```python
from build123d import *

# Parameters (mm, degrees)
F0_W     = 505
F0_H     = 250
F1_DEPTH = 40
F2_W     = 70
F2_H     = 20
F3_DEPTH = 3
F4_R     = 5
F5_DEPTH = 110


with BuildPart() as f1:
    # F0 (on Top) → F1 (new body)
    with BuildSketch(Plane.XY):
        Rectangle(F0_W, F0_H)
    extrude(amount=F1_DEPTH)

    # F2 (on face) → F3 (cut)
    with BuildSketch(Plane.XZ.offset(125)):
        with Locations((155, 20)):
            Rectangle(F2_W, F2_H)
        with Locations((-155, 20)):
            Rectangle(F2_W, F2_H)
    extrude(amount=-F3_DEPTH, mode=Mode.SUBTRACT)

    # F4 (on face) → F5 (cut)
    with BuildSketch(Plane.XZ.offset(122)):
        with Locations((-155, 20)):
            Circle(F4_R)
        with Locations((155, 20)):
            Circle(F4_R)
    extrude(amount=-F5_DEPTH, mode=Mode.SUBTRACT)


solid = f1.part
```
Design review of the part built by this model. Coordinates are the model's own, in mm. A direction names the side the tool comes from. Round coordinates to 2 decimals unless told otherwise and drop trailing zeros. Write each loop counter-clockwise with the first axis right and the second up, starting at its lowest first coordinate (ties: lowest second). Pieces come first, ordered by that corner, then holes.
Item 1: For faces 1 (the flat face through (-4, 2, 40)), 2 (the cylindrical face through (151, -68, 17)), list the 3-axis set-ups (+Z, -Z, +X, -X, +Y, -Y) from which the entire face can be reached by the end or side of a thin tool; tool diameter is ignored.
Item 2: Clearance check with flat-ended pins moving along their axes: pin 1 Ø9 at (x, z) = (-155, 20) entering from -Y; pin 2 Ø0.9 at (x, y) = (-164, -123) entering from -Z. State where each tip first meets the part, or that it passes through.
Item 3: The part is to be moulded in two halves that separate along X. For faces 3 (the flat face through (-252.5, -2, 20)), 4 (the cylindrical face through (-159, -68, 17)), 5 (the flat face through (-4, -125, 20)), say which applies: +X half, -X half, draft (parallel to the pull), parting line (faces both ways), or undercut.
Item 4: We need section A-A on x = -155. Write out the cut boundary in (y, z).
Item 5: For probe 1 along Z at (x, y) = (-155, -50); probe 2 along X at (y, z) = (-34, 21.5); probe 3 along Y at (x, z) = (-136.5, 12.5), list the stretches that pass through material, from the lowest coordinate up.
Item 6: We need section B-B on z = 20. Write out the cut boundary in (x, y), and give its area (3 significant figures).
Returned:
1. face 1: +Z, +X, -X, +Y, -Y
1. face 2: -Y
2. pin 1: stops at y = -12
2. pin 2: stops at z = 0
3. face 3: -X half
3. face 4: undercut
3. face 5: draft
4. outline: (-125, 0) - (125, 0) - (125, 40) - (-125, 40) - (-125, 30) - (-122, 30) - (-122, 25) - (-12, 25) - (-12, 15) - (-122, 15) - (-122, 10) - (-125, 10) - close
5. probe 1: z = 0 to 15, 25 to 40
5. probe 2: x = -252.5 to -159.77, -150.23 to 150.23, 159.77 to 252.5
5. probe 3: y = -122 to 125
6. outline: (-252.5, -125) - (-190, -125) - (-190, -122) - (-160, -122) - (-160, -12) - (-150, -12) - (-150, -122) - (-120, -122) - (-120, -125) - (120, -125) - (120, -122) - (150, -122) - (150, -12) - (160, -12) - (160, -122) - (190, -122) - (190, -125) - (252.5, -125) - (252.5, 125) - (-252.5, 125) - close
6. area: 124,000 mm2
